Work out the finished part from the listing and answer in its coordinate system (mm). Face numbers are marked on the shaded views. A direction names the side the tool comes from. Round coordinates to 2 decimals unless told otherwise and drop trailing zeros. Loops run counter-clockwise (first coordinate to the right, second up) from the corner with the lowest first, then second, coordinate; pieces in that order, holes last. Notation, with made-up numbers: (-5, 31) - (29, 31) arc R17 cw to (29, 58) - close; hole circle Ø2 at (86.5, 28). An arc over 180 degrees is marked (long way). Return JSON: item names as keys, results as strings.
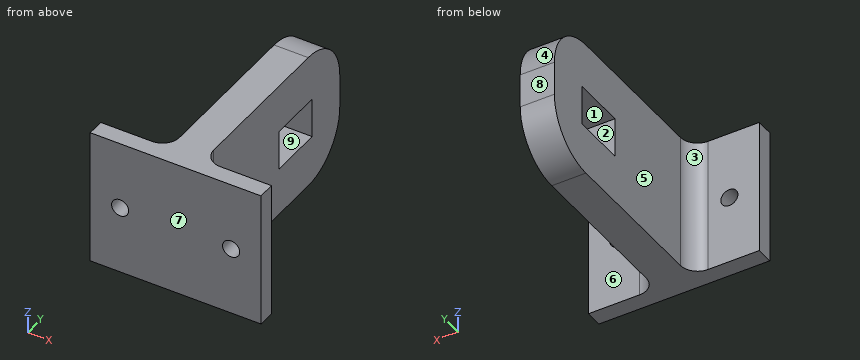
from build123d import *

# Parameters (mm, degrees)
SKETCH1_W           = 50.8
SKETCH1_H           = 88.9
SKETCH1_W_2         = 14.859
SKETCH1_H_2         = 19.939
BOSS_EXTRUDE1_DEPTH = 6.35
SKETCH2_W           = 50.8
SKETCH2_H           = 6.35
BOSS_EXTRUDE2_DEPTH = 31.75
FILLET1_R           = 6.35
SKETCH3_R           = 3.175
CUT_EXTRUDE1_DEPTH  = 93.020242338
FILLET2_R           = 19.05


with BuildPart() as part:
    # Sketch1 → Boss-Extrude1 (new, symmetric)
    with BuildSketch(Plane(origin=(0, 0, 0), x_dir=(0, 0, -1), z_dir=(1, 0, 0))):
        Rectangle(SKETCH1_W, SKETCH1_H)
        with Locations((0, 17.78)):
            Rectangle(SKETCH1_W_2, SKETCH1_H_2, mode=Mode.SUBTRACT)
    extrude(amount=BOSS_EXTRUDE1_DEPTH, both=True)

    # Sketch2 → Boss-Extrude2 (add, symmetric)
    with BuildSketch(Plane(origin=(0, 0, 0), x_dir=(0, 0, -1), z_dir=(1, 0, 0))):
        with Locations((0, -41.275)):
            Rectangle(SKETCH2_W, SKETCH2_H)
    extrude(amount=BOSS_EXTRUDE2_DEPTH, both=True)

    # Fillet1
    fillet1_edges = [part.edges().sort_by_distance(p)[0] for p in [
        (6.35, -38.1, 0),
        (-6.35, -38.1, 0),
    ]]
    fillet(fillet1_edges, radius=FILLET1_R)

    # Sketch3 → Cut-Extrude1 (cut, through all)
    with BuildSketch(Plane(origin=(0, -38.1, 0), x_dir=(1, 0, 0), z_dir=(0, 1, 0))):
        with Locations(Location((20.6375, 0, 0), (0, 0, 270))):
            Circle(SKETCH3_R)
    cut_extrude1 = extrude(amount=-CUT_EXTRUDE1_DEPTH, mode=Mode.SUBTRACT)

    # Mirror1: Cut-Extrude1 across plane
    add(cut_extrude1.mirror(Plane(origin=(0, 0, 0), x_dir=(0, 0, 1), z_dir=(1, 0, 0))), mode=Mode.SUBTRACT)

    # Fillet2
    fillet2_edges = [part.edges().sort_by_distance(p)[0] for p in [
        (0, 44.45, 25.4),
        (0, 44.45, -25.4),
    ]]
    fillet(fillet2_edges, radius=FILLET2_R)


solid = part.part
1) Flat-ended cylindrical pins translate along their axes: pin 1 (9.5 mm diameter, centred on x = 23.5, z = 8, fed in from +Y); pin 2 (8 mm diameter, centred on y = 35, z = -17, fed in from +X); pin 3 (10 mm diameter, centred on y = 35, z = -6, fed in from -X). Find the tip coordinate at first contact, or state that the pin passes through.
Verdict:
{"pin 1": "stops at y = -38.1", "pin 2": "stops at x = 6.35", "pin 3": "stops at x = -6.35"}
2) Determine the mould class of the marked faces 1, 2, 3 and 4 for opening direction Z: pulls with the +Z half, pulls with the -Z half, needs draft (parallel to the pull), parting line crosses it, or undercut.
Verdict:
{"face 1": "undercut", "face 2": "undercut", "face 3": "needs draft", "face 4": "pulls with the +Z half"}
3) Section A-A (y = 14) is taken. Give the vertices of the cut face in (x, z).
Verdict:
{"outline": "(-6.35, -25.4) - (6.35, -25.4) - (6.35, -7.43) - (-6.35, -7.43) - close; (-6.35, 7.43) - (6.35, 7.43) - (6.35, 25.4) - (-6.35, 25.4) - close"}
4) A tool of negligible diameter and unlimited length cuts with its end or side. For the marked faces 5, 6, 7, 8 and 9, from which of +Z, -Z, +X, -X, +Y, -Y can it reach the whole face along a straight path? Write none if from no direction.
Verdict:
{"face 5": "+Z, -Z, -X, +Y", "face 6": "+Z, -Z, +X, +Y", "face 7": "+Z, -Z, +X, -X, -Y", "face 8": "+Z, -Z, +X, -X, +Y", "face 9": "+X, -X"}
5) Find the intervals of material crossed by L1, parallel to X at y = -41, z = 0; L2, parallel to X at y = -5, z = 20.5; L3, parallel to Y at x = 24.5, z = 0, in increasing order.
Verdict:
{"L1": "x = -31.75 to -23.81, -17.46 to 17.46, 23.81 to 31.75", "L2": "x = -6.35 to 6.35", "L3": "y = -44.45 to -38.1"}
6) Section C-C (x = 5) is taken. Give the vertices of the cut face in (y, z), and give its area (3 significant figures).
Verdict:
{"outline": "(-44.45, -25.4) - (25.4, -25.4) arc R19.05 ccw to (44.45, -6.35) - (44.45, 6.35) arc R19.05 ccw to (25.4, 25.4) - (-44.45, 25.4) - close; hole (7.81, -7.43) - (27.75, -7.43) - (27.75, 7.43) - (7.81, 7.43) - close", "area": "4,060 mm2"}
7) Section B-B (z = 0) is taken. Give the vertices of the cut face in (x, y), and give its area (3 significant figures).
Verdict:
{"outline": "(-31.75, -44.45) - (-23.81, -44.45) - (-23.81, -38.1) - (-31.75, -38.1) - close; (-17.46, -44.45) - (17.46, -44.45) - (17.46, -38.1) - (12.7, -38.1) arc R6.35 cw to (6.35, -31.75) - (6.35, 7.81) - (-6.35, 7.81) - (-6.35, -31.75) arc R6.35 cw to (-12.7, -38.1) - (-17.46, -38.1) - close; (-6.35, 27.75) - (6.35, 27.75) - (6.35, 44.45) - (-6.35, 44.45) - close; (23.81, -44.45) - (31.75, -44.45) - (31.75, -38.1) - (23.81, -38.1) - close", "area": "1,140 mm2"}
8) Section D-D (z = -12) is taken. Give the vertices of the cut face in (x, y).
Verdict:
{"outline": "(-31.75, -44.45) - (31.75, -44.45) - (31.75, -38.1) - (12.7, -38.1) arc R6.35 cw to (6.35, -31.75) - (6.35, 43.59) - (-6.35, 43.59) - (-6.35, -31.75) arc R6.35 cw to (-12.7, -38.1) - (-31.75, -38.1) - close"}
